Input: part model. Units: mm. Frame: model coordinates. Face numbers are marked on the shaded views. A direction names the side the tool comes from. Coordinates: 2 decimals unless noted, no trailing zeros. Write each loop counter-clockwise with the first axis right and the second up, starting at its lowest first coordinate (ties: lowest second). Pieces come first, ordered by that corner, then holes. Notation, with made-up numbers: (55, 63) - (59, 63) arc R24 cw to (59, 76) - close; hole circle Ø6 at (8, 2). An arc over 180 degrees is marked (long way). Put each result on its own line as item: value. Start each with the question number.
1. Cut plane D-D, the plane z = 2.25. Return loops of the section in (x, y).
2. Cut plane C-C, the plane x = 22.5. Return loops of the section in (y, z), and give its area (3 significant figures).
3. Line query: line 1 (Z direction, x = 11, y = -24.5); line 2 (Z direction, x = 31, y = 2); line 3 (Y direction, x = 9, z = 1). Output: solid intervals per line, ascending.
4. Pin query (flat end, axial travel): pin 1 (5 mm diameter, centred on x = 17, y = 1, fed in from +Z); pin 2 (6 mm diameter, centred on y = -21, z = 12.5, fed in from -X); pin 3 (5 mm diameter, centred on x = 3, z = 19, fed in from -Y). Return the tip coordinate at first contact, or that it passes through.
5. Access query for the marked faces 4, 5, 6, 7 and 8. Directions: +Z, -Z, +X, -X, +Y, -Y. A direction counts if a zero-diameter tool reaches every point of the face in a straight line with its end or side. Return the directions, or none.
6. Pull-direction query (X, two-part tool) for the marked faces 1, 2 and 3; classes: released by +X, released by -X, zero draft, split by the parting line, or undercut.
7. Cut plane B-B, the plane z = 12.75. Return loops of the section in (x, y), and give its area (3 significant figures).
8. Cut plane A-A, the plane y = -2. Return loops of the section in (x, z), and give its area (3 significant figures).
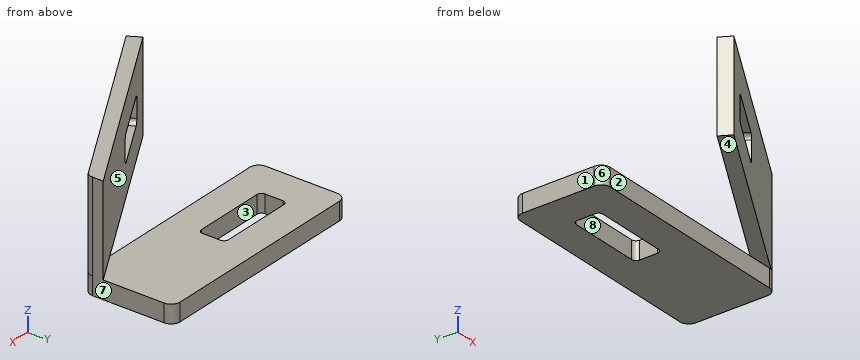
from build123d import *

# Parameters (mm, degrees)
BOSS_EXTRU_1_DEPTH      = 4
ENL_V_MAT_EXTRU_1_DEPTH = 50
BOSS_EXTRU_2_DEPTH      = 20
ENL_V_MAT_EXTRU_2_REACH = 47.943


with BuildPart() as part:
    # Esquisse1 → Boss.-Extru.1 (new body)
    with BuildSketch(Plane.XY):
        with BuildLine():
            Line((-11.273273273, 8.708708709), (34.726726727, 8.708708709))
            ThreePointArc((34.726726727, 8.708708709), (36.140940289, 8.122922271), (36.726726727, 6.708708709))
            Line((36.726726727, 6.708708709), (36.726726727, -9.291291291))
            ThreePointArc((36.726726727, -9.291291291), (36.140940289, -10.705504854), (34.726726727, -11.291291291))
            Line((34.726726727, -11.291291291), (-11.273273273, -11.291291291))
            ThreePointArc((-11.273273273, -11.291291291), (-12.687486836, -10.705504854), (-13.273273273, -9.291291291))
            Line((-13.273273273, -9.291291291), (-13.273273273, 6.708708709))
            ThreePointArc((-13.273273273, 6.708708709), (-12.687486836, 8.122922271), (-11.273273273, 8.708708709))
        make_face()
    extrude(amount=BOSS_EXTRU_1_DEPTH)

    # Esquisse3 → Enlèv. mat.-Extru.1 (cut)
    with BuildSketch(Plane.XY.offset(4)):
        with BuildLine():
            Line((-4.273273273, 1.708708709), (11.726726727, 1.708708709))
            ThreePointArc((11.726726727, 1.708708709), (12.433833508, 1.41581549), (12.726726727, 0.708708709))
            Line((12.726726727, 0.708708709), (12.726726727, -3.291291291))
            ThreePointArc((12.726726727, -3.291291291), (12.433833508, -3.998398072), (11.726726727, -4.291291291))
            Line((11.726726727, -4.291291291), (-4.273273273, -4.291291291))
            ThreePointArc((-4.273273273, -4.291291291), (-4.980380054, -3.998398072), (-5.273273273, -3.291291291))
            Line((-5.273273273, -3.291291291), (-5.273273273, 0.708708709))
            ThreePointArc((-5.273273273, 0.708708709), (-4.980380054, 1.41581549), (-4.273273273, 1.708708709))
        make_face()
    extrude(amount=-ENL_V_MAT_EXTRU_1_DEPTH, mode=Mode.SUBTRACT)

    # Esquisse4 → Boss.-Extru.2 (add)
    with BuildSketch(Plane.XY.offset(4)):
        with BuildLine():
            Line((36.141746361, -10.704698322), (-7.159396677, -35.704918553))
            Line((-7.159396677, -35.704918553), (-8.659409891, -33.10684997))
            Line((-8.659409891, -33.10684997), (36.726726727, -6.902843996))
            Line((36.726726727, -6.902843996), (36.726726727, -9.291291291))
            ThreePointArc((36.726726727, -9.291291291), (36.5747039, -10.056131383), (36.141746361, -10.704698322))
        make_face()
    extrude(amount=BOSS_EXTRU_2_DEPTH)

    # Esquisse5 → Enlèv. mat.-Extru.2 (cut, up to next)
    with BuildSketch(Plane(origin=(12.170880133, -21.08033516, 0), x_dir=(0.8660228607631385, 0.500004404616229, 0), z_dir=(-0.500004404616229, 0.8660228607631385, 0)), mode=Mode.PRIVATE) as enl_v_mat_extru_2_sk1:
        with BuildLine():
            Line((-15.052817734, -11), (-1.632555066, -11))
            ThreePointArc((-1.632555066, -11), (-0.925448284, -11.292893219), (-0.632555066, -12))
            Line((-0.632555066, -12), (-0.632555066, -16))
            ThreePointArc((-0.632555066, -16), (-0.925448284, -16.707106781), (-1.632555066, -17))
            Line((-1.632555066, -17), (-15.052817734, -17))
            ThreePointArc((-15.052817734, -17), (-15.759924515, -16.707106781), (-16.052817734, -16))
            Line((-16.052817734, -16), (-16.052817734, -12))
            ThreePointArc((-16.052817734, -12), (-15.759924515, -11.292893219), (-15.052817734, -11))
        make_face()
    enl_v_mat_extru_2_tool1 = extrude(enl_v_mat_extru_2_sk1.sketch, amount=-ENL_V_MAT_EXTRU_2_REACH, mode=Mode.PRIVATE) & part.part
    add(enl_v_mat_extru_2_tool1.solids().sort_by_distance((4.945923, -25.251715, 14))[0], mode=Mode.SUBTRACT)


solid = part.part
Report:
1. outline: (-13.27, -9.29) arc R2 ccw to (-11.27, -11.29) - (34.73, -11.29) arc R2 ccw to (36.73, -9.29) - (36.73, 6.71) arc R2 ccw to (34.73, 8.71) - (-11.27, 8.71) arc R2 ccw to (-13.27, 6.71) - close; hole (-5.27, -3.29) arc R1 ccw to (-4.27, -4.29) - (11.73, -4.29) arc R1 ccw to (12.73, -3.29) - (12.73, 0.71) arc R1 ccw to (11.73, 1.71) - (-4.27, 1.71) arc R1 ccw to (-5.27, 0.71) - close
2. outline: (-18.58, 4) - (-15.12, 4) - (-15.12, 24) - (-18.58, 24) - close; (-11.29, 0) - (8.71, 0) - (8.71, 4) - (-11.29, 4) - close
2. area: 149 mm^2
3. line 1: z = 4 to 11, 17 to 24
3. line 2: z = 0 to 4
3. line 3: y = -11.29 to -4.29, 1.71 to 8.71
4. pin 1: stops at z = 4
4. pin 2: stops at x = 7.81
4. pin 3: stops at y = -31.28
5. face 4: -Z, +X, -X, -Y
5. face 5: +Z, -X, +Y
5. face 6: +Z, -Z, -X, -Y
5. face 7: +Z, -Z, +X, +Y, -Y
5. face 8: +Z, -Z
6. face 1: released by -X
6. face 2: zero draft
6. face 3: undercut
7. outline: (-8.66, -33.11) - (-7.16, -35.7) - (-0.23, -31.7) - (-1.73, -29.11) - close; (11.62, -21.4) - (13.12, -23.99) - (36.14, -10.7) arc R2 ccw to (36.73, -9.29) - (36.73, -6.9) - close
7. area: 108 mm^2
8. outline: (-13.27, 0) - (-5.27, 0) - (-5.27, 4) - (-13.27, 4) - close; (12.73, 0) - (36.73, 0) - (36.73, 4) - (12.73, 4) - close
8. area: 128 mm^2
